Design review of the part built by this model. Coordinates are the model's own, in mm. Face numbers are marked on the shaded views. A direction names the side the tool comes from. Round coordinates to 2 decimals unless told otherwise and drop trailing zeros. Loops run counter-clockwise (first coordinate to the right, second up) from the corner with the lowest first, then second, coordinate; pieces in that order, holes last. Notation, with made-up numbers: M 69.5,12 L 91.5,12 A11 ccw 91.5,24 Z; hole C 39,52 d4. An arc over 180 degrees is marked long. Use a Markdown table: item, result.
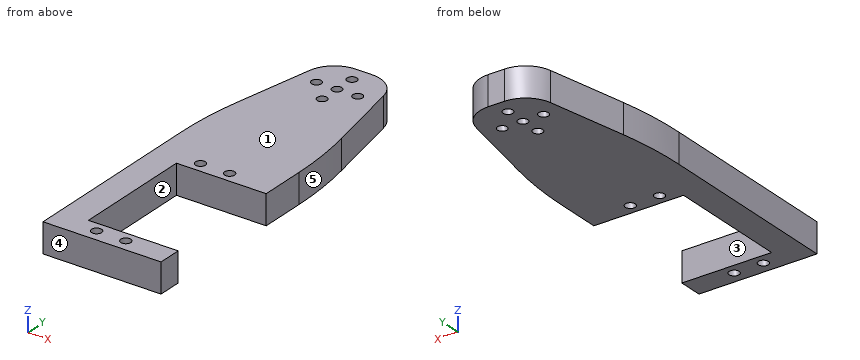
from build123d import *

# Parameters (mm, degrees)
SKETCH2_W           = 40
SKETCH2_H           = 122.5
BOSS_EXTRUDE1_DEPTH = 10
SKETCH3_R           = 1.7
SKETCH3_W           = 20.8
SKETCH3_H           = 41.2
CUT_EXTRUDE3_DEPTH  = 130.252659547
SKETCH4_R           = 1.65
CUT_EXTRUDE4_DEPTH  = 130.252659547
SKETCH5_W           = 30.4
SKETCH5_H           = 41.2
SKETCH5_W_2         = 9
SKETCH5_H_2         = 52.5
CUT_EXTRUDE5_DEPTH  = 130.252659547
DRAFT11_DEPTH       = 10
FILLET4_R           = 120
FILLET5_R           = 10


# Read off the part's stored shape, not the designer's step: Draft11
with BuildPart() as part:
    # Sketch2 → Boss-Extrude1 (new body)
    with BuildSketch(Plane.XY):
        with Locations((-20, 61.25)):
            Rectangle(SKETCH2_W, SKETCH2_H)
    extrude(amount=BOSS_EXTRUDE1_DEPTH)

    # Sketch3 → Cut-Extrude3 (cut, through all)
    with BuildSketch(Plane.XY):
        with Locations((-24.95, 4.3)):
            Circle(SKETCH3_R)
        with Locations((-15.05, 4.3)):
            Circle(SKETCH3_R)
        with Locations(Location((-15.05, 52.9, 0), (0, 0, 180))):
            Circle(SKETCH3_R)
        with Locations(Location((-24.95, 52.9, 0), (0, 0, 180))):
            Circle(SKETCH3_R)
        with Locations((-20, 28.6)):
            Rectangle(SKETCH3_W, SKETCH3_H)
    extrude(amount=CUT_EXTRUDE3_DEPTH, mode=Mode.SUBTRACT)

    # Sketch4 → Cut-Extrude4 (cut, through all)
    with BuildSketch(Plane.XY.offset(10)):
        with Locations((-20, 110)):
            Circle(SKETCH4_R)
        with Locations((-27, 110)):
            Circle(SKETCH4_R)
        with Locations((-20, 117)):
            Circle(SKETCH4_R)
        with Locations((-13, 110)):
            Circle(SKETCH4_R)
        with Locations((-20, 103)):
            Circle(SKETCH4_R)
    extrude(amount=-CUT_EXTRUDE4_DEPTH, mode=Mode.SUBTRACT)

    # Sketch5 → Cut-Extrude5 (cut, through all)
    with BuildSketch(Plane.XY.offset(10)):
        with Locations((-15.2, 28.6)):
            Rectangle(SKETCH5_W, SKETCH5_H)
        with Locations((-35.5, 96.25)):
            Rectangle(SKETCH5_W_2, SKETCH5_H_2)
        with Locations((-4.5, 96.25)):
            Rectangle(SKETCH5_W_2, SKETCH5_H_2)
    extrude(amount=-CUT_EXTRUDE5_DEPTH, mode=Mode.SUBTRACT)

    # Draft11 outline → Draft11 (add)
    with BuildSketch(Plane.XY):
        Polygon((0, 70), (0, 76.199013856), (-9, 122.5), (-9, 70), align=None)
        Polygon((-31, 70), (-31, 122.5), (-40, 76.199013856), (-40, 70), align=None)
    extrude(amount=DRAFT11_DEPTH)

    # Fillet4
    fillet4_edges = [part.edges().sort_by_distance(p)[0] for p in [
        (0, 76.199013856, 5),
        (-40, 76.199013856, 5),
    ]]
    fillet(fillet4_edges, radius=FILLET4_R)

    # Fillet5
    fillet5_edges = [part.edges().sort_by_distance(p)[0] for p in [
        (-9, 122.5, 5),
        (-31, 122.5, 5),
    ]]
    fillet(fillet5_edges, radius=FILLET5_R)


solid = part.part
1. Wall thickness on line 1 along Y through (x, z) = (-20, 5); line 2 along X through (y, z) = (52.9, 7); line 3 along Y through (x, z) = (-25.5, 1.25): over which ranges is each line inside the solid? List them lowest first. Write a range as from..to.
Check values:
| item | result |
|---|---|
| line 1 | y = 0..8, 49.2..101.35, 104.65..108.35, 111.65..115.35, 118.65..122.5 |
| line 2 | x = -40..-26.65, -23.25..-16.75, -13.35..0 |
| line 3 | y = 0..2.69, 5.91..8, 49.2..51.29, 54.51..109.31, 110.69..122.12 |
2. The part is to be moulded in two halves that separate along Y. For the marked faces 3, 4 and 5, say which applies: pulls with the +Y half, pulls with the -Y half, needs draft (parallel to the pull), parting line crosses it, or undercut.
Check values:
| item | result |
|---|---|
| face 3 | undercut |
| face 4 | pulls with the -Y half |
| face 5 | pulls with the +Y half |
3. Take a section at C-C on y = 103. Give the boundary of the cut face in (x, z).
Check values:
| item | result |
|---|---|
| outline | M -34.79,0 L -21.65,0 L -21.65,10 L -34.79,10 Z; M -18.35,0 L -5.21,0 L -5.21,10 L -18.35,10 Z |
4. Insertion check: pin 1 (3 mm diameter, centred on x = -15.05, y = 52.9, fed in from -Z); pin 2 (5 mm diameter, centred on y = 99, z = 2.5, fed in from +X); pin 3 (4 mm diameter, centred on x = -10.5, z = 6.5, fed in from +Y). Each pin has a flat end and moves straight along its axis. Give the tip position at first contact, or say it passes through.
Check values:
| item | result |
|---|---|
| pin 1 | passes through |
| pin 2 | stops at x = -3.95 |
| pin 3 | stops at y = 121.3 |
5. Take a section at D-D on x = -5. Give the boundary of the cut face in (y, z).
Check values:
| item | result |
|---|---|
| outline | M 0,0 L 8,0 L 8,10 L 0,10 Z; M 49.2,0 L 101.92,0 L 101.92,10 L 49.2,10 Z |
6. Machinability: for the marked faces 1 and 2, which of the approach directions +Z, -Z, +X, -X, +Y, -Y give a long, thin tool a straight path to every point of the face, cutting with its end or side? Answer none if there is none.
Check values:
| item | result |
|---|---|
| face 1 | +Z, +X, -X, +Y, -Y |
| face 2 | +Z, -Z, +X |
7. Take a section at A-A on x = -20. Give the boundary of the cut face in (y, z).
Check values:
| item | result |
|---|---|
| outline | M 0,0 L 8,0 L 8,10 L 0,10 Z; M 49.2,0 L 101.35,0 L 101.35,10 L 49.2,10 Z; M 104.65,0 L 108.35,0 L 108.35,10 L 104.65,10 Z; M 111.65,0 L 115.35,0 L 115.35,10 L 111.65,10 Z; M 118.65,0 L 122.5,0 L 122.5,10 L 118.65,10 Z |
8. Take a section at B-B on z = 1.5. Count the separate pieces of the cut face and the enclosed holes in it, and give its area (3 significant figures).
Check values:
| item | result |
|---|---|
| separate pieces | 1 |
| enclosed holes | 9 |
| area | 3,120 mm² |
